The model under review builds one solid part; all positions refer to its coordinate system, in mm. Coordinates: 2 decimals unless noted, no trailing zeros. Order: outer loops, then holes, each group sorted by start corner. A loop starts at its lowest first (then second) coordinate and runs counter-clockwise, first axis right, second up. Notation, with made-up numbers: (-8, 77) -> (23, 77) arc R29 cw to (23, 106) -> close; hole circle Ø8 at (40.5, 13.5). An arc over 180 degrees is marked (long way). Use one line per item in the form item = value.
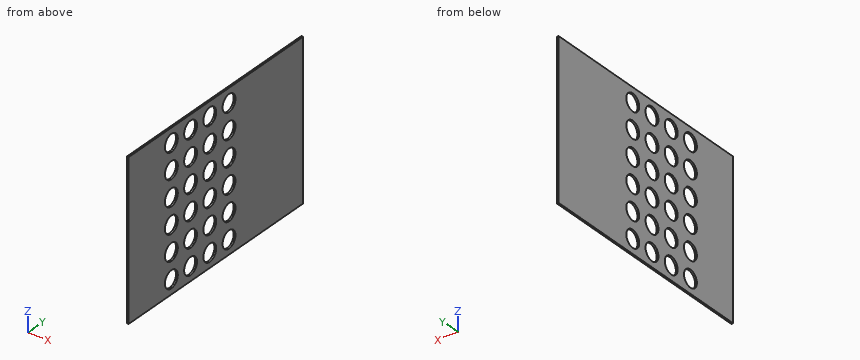
from build123d import *

# Parameters (mm, degrees)
BOX005_W         = 6.35
BOX005_H         = 150
BOX005_DEPTH     = 550.2
BOX004_W         = 6.35
BOX004_H         = 297
BOX004_DEPTH     = 550.2
SKETCH002_R      = 30.15
PAD001_DEPTH     = 200
ARRAY001_X_COUNT = 2
ARRAY001_X_PITCH = 1
ARRAY001_Y_COUNT = 4
ARRAY001_Y_PITCH = 90
ARRAY001_Z_COUNT = 6
ARRAY001_Z_PITCH = 90
BOX001_W         = 6.35
BOX001_H         = 370.3
BOX001_DEPTH     = 550.2


with BuildPart() as obj1:
    # Box005 → Box005 (new body)
    with BuildSketch(Plane(origin=(0, -999, -44), x_dir=(1, 0, 0), z_dir=(0, 0, 1))):
        with Locations((3.175, 75)):
            Rectangle(BOX005_W, BOX005_H)
    extrude(amount=BOX005_DEPTH)


with BuildPart() as cubo004:
    # Box004 → Box004 (new body)
    with BuildSketch(Plane(origin=(0, -478.7, -44), x_dir=(1, 0, 0), z_dir=(0, 0, 1))):
        with Locations((3.175, 148.5)):
            Rectangle(BOX004_W, BOX004_H)
    extrude(amount=BOX004_DEPTH)


with BuildPart() as obj2:
    # Sketch002 → Pad001 (new body)
    with BuildSketch(Plane.YZ):
        Circle(SKETCH002_R)
    extrude(amount=PAD001_DEPTH)


with BuildPart() as obj2_1:
    # Body001 placement: moved
    add(obj2.part.moved(Location((-418, 209, 0))))

    # Array001 X: obj2_2


with BuildPart() as obj2_2:
    add(obj2_1.part)
    with Locations(*[(i * ARRAY001_X_PITCH, 0, 0) for i in range(1, ARRAY001_X_COUNT)]):
        add(obj2_1.part)

    # Array001 Y: obj2_4


with BuildPart() as obj2_3:
    add(obj2_2.part)
    with Locations(*[(0, i * ARRAY001_Y_PITCH, 0) for i in range(1, ARRAY001_Y_COUNT)]):
        add(obj2_2.part)

    # Array001 Z: obj2 ×6


with BuildPart() as obj2_4:
    add(obj2_3.part)
    with Locations(*[(0, 0, i * ARRAY001_Z_PITCH) for i in range(1, ARRAY001_Z_COUNT)]):
        add(obj2_3.part)


with BuildPart() as obj2_5:
    # Array001 placement: moved
    add(obj2_4.part.moved(Location((228.35, -1007.85, 6.05))))


with BuildPart() as placa_portatubo1:
    # Box001 → Box001 (new body)
    with BuildSketch(Plane(origin=(0, -849, -44), x_dir=(1, 0, 0), z_dir=(0, 0, 1))):
        with Locations((3.175, 185.15)):
            Rectangle(BOX001_W, BOX001_H)
    extrude(amount=BOX001_DEPTH)

    # Cut: cut obj2
    add(obj2_5.part, mode=Mode.SUBTRACT)

    # Fusion: union Cubo004
    add(cubo004.part)

    # Fusion001: union obj1
    add(obj1.part)


solid = placa_portatubo1.part
Item 1: We need section D-D (z = 202.5). Write out the cut boundary in (x, y), plus the area to 3 significant figures.
Results found:
outline = (0, -999) -> (6.35, -999) -> (6.35, -824.12) -> (0, -824.12) -> close; (0, -773.58) -> (6.35, -773.58) -> (6.35, -734.12) -> (0, -734.12) -> close; (0, -683.58) -> (6.35, -683.58) -> (6.35, -644.12) -> (0, -644.12) -> close; (0, -593.58) -> (6.35, -593.58) -> (6.35, -554.12) -> (0, -554.12) -> close; (0, -503.58) -> (6.35, -503.58) -> (6.35, -181.7) -> (0, -181.7) -> close
area = 3,910 mm²
Item 2: We need section A-A (z = 366.05). Write out the cut boundary in (x, y).
Results found:
outline = (0, -999) -> (6.35, -999) -> (6.35, -829) -> (0, -829) -> close; (0, -768.7) -> (6.35, -768.7) -> (6.35, -739) -> (0, -739) -> close; (0, -678.7) -> (6.35, -678.7) -> (6.35, -649) -> (0, -649) -> close; (0, -588.7) -> (6.35, -588.7) -> (6.35, -559) -> (0, -559) -> close; (0, -498.7) -> (6.35, -498.7) -> (6.35, -181.7) -> (0, -181.7) -> close
Item 3: We need section B-B (y = -708.85). Write out the cut boundary in (x, z).
Results found:
outline = (0, -44) -> (6.35, -44) -> (6.35, -24.1) -> (0, -24.1) -> close; (0, 36.2) -> (6.35, 36.2) -> (6.35, 65.9) -> (0, 65.9) -> close; (0, 126.2) -> (6.35, 126.2) -> (6.35, 155.9) -> (0, 155.9) -> close; (0, 216.2) -> (6.35, 216.2) -> (6.35, 245.9) -> (0, 245.9) -> close; (0, 306.2) -> (6.35, 306.2) -> (6.35, 335.9) -> (0, 335.9) -> close; (0, 396.2) -> (6.35, 396.2) -> (6.35, 425.9) -> (0, 425.9) -> close; (0, 486.2) -> (6.35, 486.2) -> (6.35, 506.2) -> (0, 506.2) -> close
Item 4: Clearance check with a flat-ended pin moving along its axis: pin 1 (8 mm diameter, centred on y = -896, z = 68.5, fed in from -X). State where the tip first meets the part, or that it passes through.
Results found:
pin_1 = 0
Item 5: To check wall thickness, follow L1, parallel to Y at x = 5, z = 6.05; L2, parallel to Y at x = 0.75, z = 163. State the ranges of each line that lie inside material, in increasing order. Write a range as from..to.
Results found:
L1 = -999..-829, -768.7..-739, -678.7..-649, -588.7..-559, -498.7..-181.7
L2 = -999..-818.29, -779.41..-728.29, -689.41..-638.29, -599.41..-548.29, -509.41..-181.7
Item 6: We need section C-C (x = 4). State how many separate pieces and enclosed holes the cut face has, plus the area to 3 significant figures.
Results found:
separate_pieces = 1
enclosed_holes = 24
area = 381,000 mm²
